Read the model definition and answer for the solid it produces. Units are mm, in the model's axes. A direction names the side the tool comes from. Give positions to 0.01 mm unless a question says otherwise; leave off trailing zeros. Write each loop counter-clockwise with the first axis right and the second up, starting at its lowest first coordinate (ties: lowest second). Pieces come first, ordered by that corner, then holes. Notation, with made-up numbers: (68.5, 68) -> (75.5, 68) arc R12 cw to (75.5, 73) -> close; hole circle Ø4 at (-27.75, -16). An arc over 180 degrees is marked (long way). Use a Markdown table: item, result.
from build123d import *

# Parameters (mm, degrees)
BOSS_EXTRUDE1_DEPTH = 8
BOSS_EXTRUDE2_DEPTH = 5
SKETCH3_W           = 25
SKETCH3_H           = 5
BOSS_EXTRUDE3_DEPTH = 8


with BuildPart() as part:
    # Sketch1 → Boss-Extrude1 (new body)
    with BuildSketch(Plane.XY):
        with BuildLine():
            Line((-12.5, 0), (-12.5, 34))
            Line((-12.5, 34), (-22.5, 34))
            Line((-22.5, 34), (-22.5, 0))
            ThreePointArc((-22.5, 0), (0, -22.5), (22.5, 0))
            Line((22.5, 0), (22.5, 34))
            Line((22.5, 34), (12.5, 34))
            Line((12.5, 34), (12.5, 0))
            ThreePointArc((12.5, 0), (0, -12.5), (-12.5, 0))
        make_face()
    extrude(amount=BOSS_EXTRUDE1_DEPTH)

    # Sketch2 → Boss-Extrude2 (add)
    with BuildSketch(Plane(origin=(0, 34, 0), x_dir=(1, 0, 0), z_dir=(0, 1, 0))):
        Polygon((-22.5, 0), (-22.5, -8.684042384), (-22.5, -16.684042384), (22.5, -16.684042384), (22.5, 0), (12.5, 0), (12.5, -8), (-12.5, -8), (-12.5, 0), align=None)
    extrude(amount=BOSS_EXTRUDE2_DEPTH)

    # Sketch3 → Boss-Extrude3 (add)
    with BuildSketch(Plane(origin=(0, 0, 8), x_dir=(-1, 0, 0), z_dir=(0, 0, -1))):
        with Locations((0, 36.5)):
            Rectangle(SKETCH3_W, SKETCH3_H)
    extrude(amount=BOSS_EXTRUDE3_DEPTH)


solid = part.part
Item 1: Each of these flat-tipped pins is pushed along its axis until it touches: P1, Ø3, axis at y = -2, z = 6.5, coming from the -X side; P2, Ø13.5, axis at x = 5, y = 6, coming from the +Z side; P3, Ø5, axis at x = -17, y = 28, coming from the +Z side; P4, Ø3, axis at x = -4, z = 3, coming from the -Y side. Where does it stop, or does it pass through?
Return value:
| item | result |
|---|---|
| P1 | x = -22.49 |
| P2 | through |
| P3 | z = 8 |
| P4 | y = -22.36 |
Item 2: For a pull along X with two mould halves and no side action, classify faces 1 (the face through (-12.5, 17, 4)), 2 (the face through (0, 36, 16.684)), 3 (the face through (22.5, 19, 5)) as +X half, -X half, draft (parallel to the pull), parting line (faces both ways), or undercut.
Return value:
| item | result |
|---|---|
| face 1 | undercut |
| face 2 | draft |
| face 3 | +X half |
Item 3: A cutting plane is placed at A-A (x = 0). Give the vertices of the cut face in (y, z).
Return value:
| item | result |
|---|---|
| outline | (-22.5, 0) -> (-12.5, 0) -> (-12.5, 8) -> (-22.5, 8) -> close; (34, 0) -> (39, 0) -> (39, 16.68) -> (34, 16.68) -> close |
Item 4: Straight lines are drawn through the part: line 1 along X through (y, z) = (11, 6); line 2 along Z through (x, y) = (-16.5, -14.5); line 3 along Y through (x, z) = (-9.5, 5.5). For each, find the intervals that lie inside material, in ascending order. Write a range as [from, to].
Return value:
| item | result |
|---|---|
| line 1 | [-22.5, -12.5], [12.5, 22.5] |
| line 2 | [0, 8] |
| line 3 | [-20.4, -8.12], [34, 39] |
Item 5: A tool of negligible diameter and unlimited length cuts with its end or side. For faces 4 (the face through (0.275, -12.497, 3.944)), 5 (the face through (-15, 6, 8)), 6 (the face through (0, 34, 10)), from which of +Z, -Z, +X, -X, +Y, -Y can it reach the whole face along a straight path? Write none if from no direction.
Return value:
| item | result |
|---|---|
| face 4 | +Z, -Z |
| face 5 | +Z, +X, -X, -Y |
| face 6 | +Z |
Item 6: A cutting plane is placed at B-B (y = 32). Give the vertices of the cut face in (x, z), then the cut area to 3 significant figures.
Return value:
| item | result |
|---|---|
| outline | (-22.5, 0) -> (-12.5, 0) -> (-12.5, 8) -> (-22.5, 8) -> close; (12.5, 0) -> (22.5, 0) -> (22.5, 8) -> (12.5, 8) -> close |
| area | 160 mm^2 |
Item 7: A cutting plane is placed at D-D (z = 11.75). Give the vertices of the cut face in (x, y).
Return value:
| item | result |
|---|---|
| outline | (-22.5, 34) -> (22.5, 34) -> (22.5, 39) -> (-22.5, 39) -> close |
Item 8: A cutting plane is placed at C-C (z = 6.5). Give the vertices of the cut face in (x, y).
Return value:
| item | result |
|---|---|
| outline | (-22.5, 0) arc R22.5 ccw to (22.5, 0) -> (22.5, 39) -> (-22.5, 39) -> close; hole (-12.5, 0) arc R12.5 ccw to (12.5, 0) -> (12.5, 34) -> (-12.5, 34) -> close |
